Work out the finished part from the listing and answer in its coordinate system (mm). Face numbers are marked on the shaded views. Round coordinates to 2 decimals unless told otherwise and drop trailing zeros. Order: outer loops, then holes, each group sorted by start corner. A loop starts at its lowest first (then second) coordinate and runs counter-clockwise, first axis right, second up. Notation, with made-up numbers: (86.5, 54) - (90.5, 54) arc R23 ccw to (90.5, 68) - close; hole circle Ø5 at (-2, -18). An arc over 180 degrees is marked (long way). Answer in a Markdown table with one row per item.
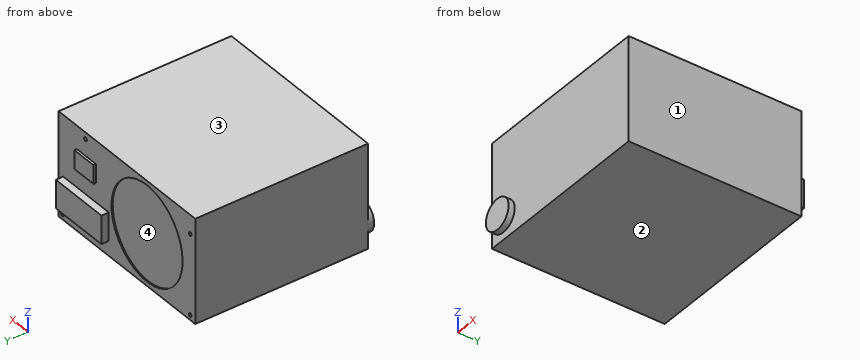
from build123d import *

# Parameters (mm, degrees)
ESQUISSE1_W             = 150
ESQUISSE1_H             = 141
BOSS_EXTRU_1_DEPTH      = 85
ESQUISSE2_W             = 21
ESQUISSE2_H             = 15.2
BOSS_EXTRU_2_DEPTH      = 2
ESQUISSE3_W             = 50
ESQUISSE3_H             = 23.11
BOSS_EXTRU_3_DEPTH      = 6
ESQUISSE4_R             = 39
ENL_V_MAT_EXTRU_1_DEPTH = 1
ESQUISSE5_R             = 1.5
ENL_V_MAT_EXTRU_2_DEPTH = 5
ESQUISSE6_R             = 12.5
BOSS_EXTRU_4_DEPTH      = 5


with BuildPart() as part:
    # Esquisse1 → Boss.-Extru.1 (new body)
    with BuildSketch(Plane.XY):
        with Locations((75, 70.5)):
            Rectangle(ESQUISSE1_W, ESQUISSE1_H)
    extrude(amount=BOSS_EXTRU_1_DEPTH)

    # Esquisse2 → Boss.-Extru.2 (add)
    with BuildSketch(Plane(origin=(0, 141, 0), x_dir=(1, 0, 0), z_dir=(0, 1, 0))):
        with Locations((119.5, -58.4)):
            Rectangle(ESQUISSE2_W, ESQUISSE2_H)
    extrude(amount=BOSS_EXTRU_2_DEPTH)

    # Esquisse3 → Boss.-Extru.3 (add)
    with BuildSketch(Plane(origin=(0, 141, 0), x_dir=(1, 0, 0), z_dir=(0, 1, 0))):
        with Locations((120, -23.555)):
            Rectangle(ESQUISSE3_W, ESQUISSE3_H)
    extrude(amount=BOSS_EXTRU_3_DEPTH)

    # Esquisse4 → Enlèv. mat.-Extru.1 (cut)
    with BuildSketch(Plane(origin=(0, 141, 0), x_dir=(1, 0, 0), z_dir=(0, 1, 0))):
        with Locations(Location((53, -42.5, 0), (0, 0, 270))):
            Circle(ESQUISSE4_R)
    extrude(amount=-ENL_V_MAT_EXTRU_1_DEPTH, mode=Mode.SUBTRACT)

    # Esquisse5 → Enlèv. mat.-Extru.2 (cut)
    with BuildSketch(Plane(origin=(0, 141, 0), x_dir=(1, 0, 0), z_dir=(0, 1, 0))):
        with Locations(Location((120.5, -79.5, 0), (0, 0, 270))):
            Circle(ESQUISSE5_R)
        with Locations(Location((5.5, -69.5, 0), (0, 0, 270))):
            Circle(ESQUISSE5_R)
        with Locations(Location((5.5, -4, 0), (0, 0, 270))):
            Circle(ESQUISSE5_R)
        with Locations(Location((146, -4, 0), (0, 0, 270))):
            Circle(ESQUISSE5_R)
    extrude(amount=-ENL_V_MAT_EXTRU_2_DEPTH, mode=Mode.SUBTRACT)

    # Esquisse6 → Boss.-Extru.4 (add)
    with BuildSketch(Plane(origin=(0, 0, 0), x_dir=(-1, 0, 0), z_dir=(0, -1, 0))):
        with Locations((-12.5, -18.5)):
            Circle(ESQUISSE6_R)
    extrude(amount=BOSS_EXTRU_4_DEPTH)


solid = part.part
1) Find section B-B, the plane z = 37. Give the vertices of the cut face in (x, y).
Filled in:
| item | result |
|---|---|
| outline | (0, 0) - (150, 0) - (150, 141) - (91.61, 141) - (91.61, 140) - (14.39, 140) - (14.39, 141) - (0, 141) - close |
2) Find section C-C, the plane z = 22. Give the vertices of the cut face in (x, y), then the cut area to 3 significant figures.
Filled in:
| item | result |
|---|---|
| outline | (0, 0) - (0.5, 0) - (0.5, -5) - (24.5, -5) - (24.5, 0) - (150, 0) - (150, 141) - (145, 141) - (145, 147) - (95, 147) - (95, 141) - (86.18, 141) - (86.18, 140) - (19.82, 140) - (19.82, 141) - (0, 141) - close |
| area | 21,500 mm^2 |
3) Each of these flat-tipped pins is pushed along its axis until it touches: pin 1 (5 mm diameter, centred on x = 5.5, z = 69.5, fed in from +Y); pin 2 (5 mm diameter, centred on x = 120.5, z = 79.5, fed in from -Y); pin 3 (5 mm diameter, centred on y = 144, z = 21, fed in from -X). Where does it stop, or does it pass through?
Filled in:
| item | result |
|---|---|
| pin 1 | stops at y = 141 |
| pin 2 | stops at y = 0 |
| pin 3 | stops at x = 95 |
4) The mould has two halves that part along Z. Classify the marked faces 1, 2, 3 and 4: released by +Z, released by -Z, zero draft, split by the parting line, or undercut.
Filled in:
| item | result |
|---|---|
| face 1 | zero draft |
| face 2 | released by -Z |
| face 3 | released by +Z |
| face 4 | undercut |
5) Find the intervals of material crossed by probe 1 along X at (y, z) = (137.9, 4); probe 2 along Z at (x, y) = (5, 138); probe 3 along X at (y, z) = (140.65, 42.5), in increasing order. Write a range as from..to.
Filled in:
| item | result |
|---|---|
| probe 1 | x = 0..4, 7..144.5, 147.5..150 |
| probe 2 | z = 0..2.59, 5.41..68.09, 70.91..85 |
| probe 3 | x = 0..14, 92..150 |
6) Find section A-A, the plane x = 137.5. Give the vertices of the cut face in (y, z), then the cut area to 3 significant figures.
Filled in:
| item | result |
|---|---|
| outline | (0, 0) - (141, 0) - (141, 12) - (147, 12) - (147, 35.11) - (141, 35.11) - (141, 85) - (0, 85) - close |
| area | 12,100 mm^2 |
